Job drawing, mm, ordinate dimensions from the low corner. One solid piece. A direction names the side the tool comes from. Give positions to 0.01 mm unless a question says otherwise; leave off trailing zeros. Order: outer loops, then holes, each group sorted by start corner. A loop starts at its lowest first (then second) coordinate and runs counter-clockwise, first axis right, second up. Notation, with made-up numbers: M -39.75,-28 L -24.75,-28 A23 cw -24.75,-11 Z; hole C 15,11.5 d9. An arc over 180 degrees is marked long. Use CSV: the item, a comma, the result in double quotes. Start each with the question number.
Item 1: Band-saw the part on A-A on z = 6. Write the cut outline in (x, y), plus the area to 3 significant figures.
Item 2: Band-saw the part on C-C on x = 19.5. Give the number of separate pieces and of enclosed holes in the cut face, plus the area to 3 significant figures.
Item 3: Which spindle directions (+Z, -Z, +X, -X, +Y, -Y) get a long thin tool onto all of the face, cutting with end or side? Do the marked faces 1 and 2. Say none if no direction does.
Item 4: Wall check: line 1 along Y through (x, z) = (44, 0.5); line 2 along Z through (x, y) = (22.5, 22.75). Give the ranges that are in metal, low to high.
Item 5: Pin check, flat tips, straight feed: P1, Ø4.5, axis at x = 12, y = 22, coming from the +Z side; P2, Ø12, axis at x = 41, z = 21, coming from the +Y side. Stop position of each tip, or through.
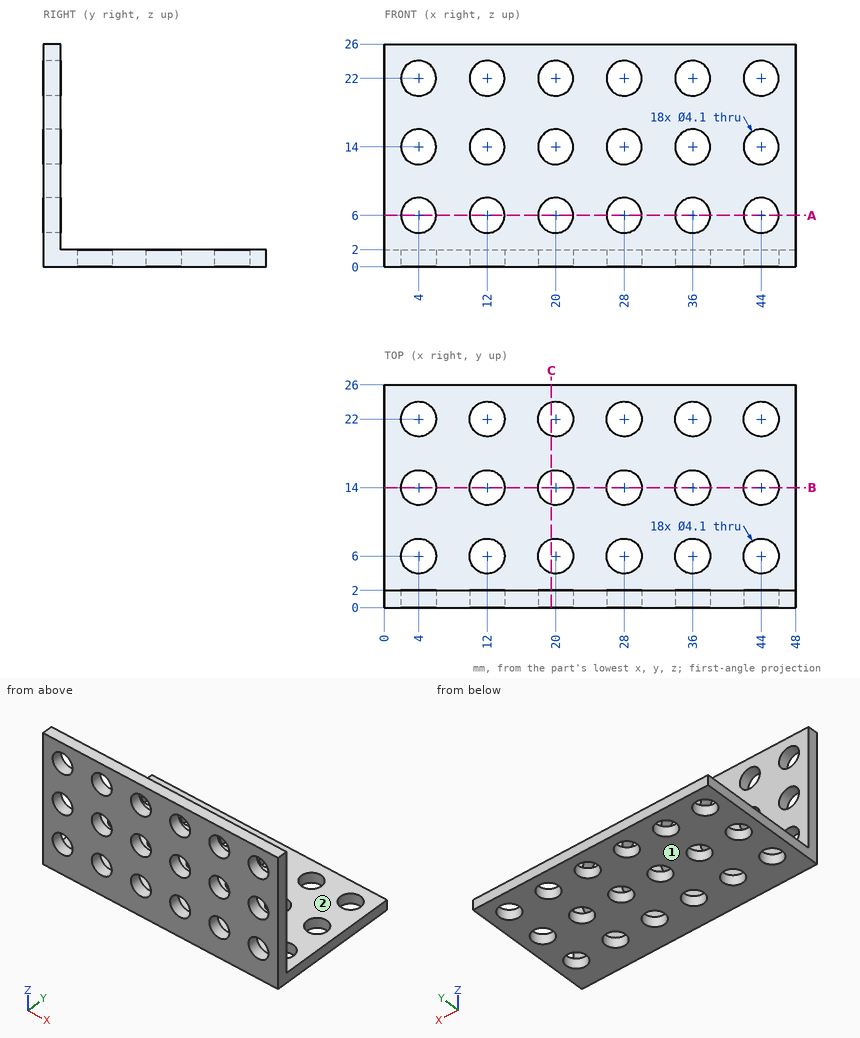
Model answer:
1,outline,"M 0,0 L 1.95,0 L 1.95,2 L 0,2 Z; M 6.05,0 L 9.95,0 L 9.95,2 L 6.05,2 Z; M 14.05,0 L 17.95,0 L 17.95,2 L 14.05,2 Z; M 22.05,0 L 25.95,0 L 25.95,2 L 22.05,2 Z; M 30.05,0 L 33.95,0 L 33.95,2 L 30.05,2 Z; M 38.05,0 L 41.95,0 L 41.95,2 L 38.05,2 Z; M 46.05,0 L 48,0 L 48,2 L 46.05,2 Z"
1,area,"46.8 mm^2"
2,separate pieces,"7"
2,enclosed holes,"0"
2,area,"52.3 mm^2"
3,face 1,"-Z, +X, -X, +Y, -Y"
3,face 2,"+Z, +X, -X, +Y"
4,line 1,"y = 0 to 3.95, 8.05 to 11.95, 16.05 to 19.95, 24.05 to 26"
4,line 2,"z = 0 to 2"
5,P1,"stops at z = 2"
5,P2,"stops at y = 2"
